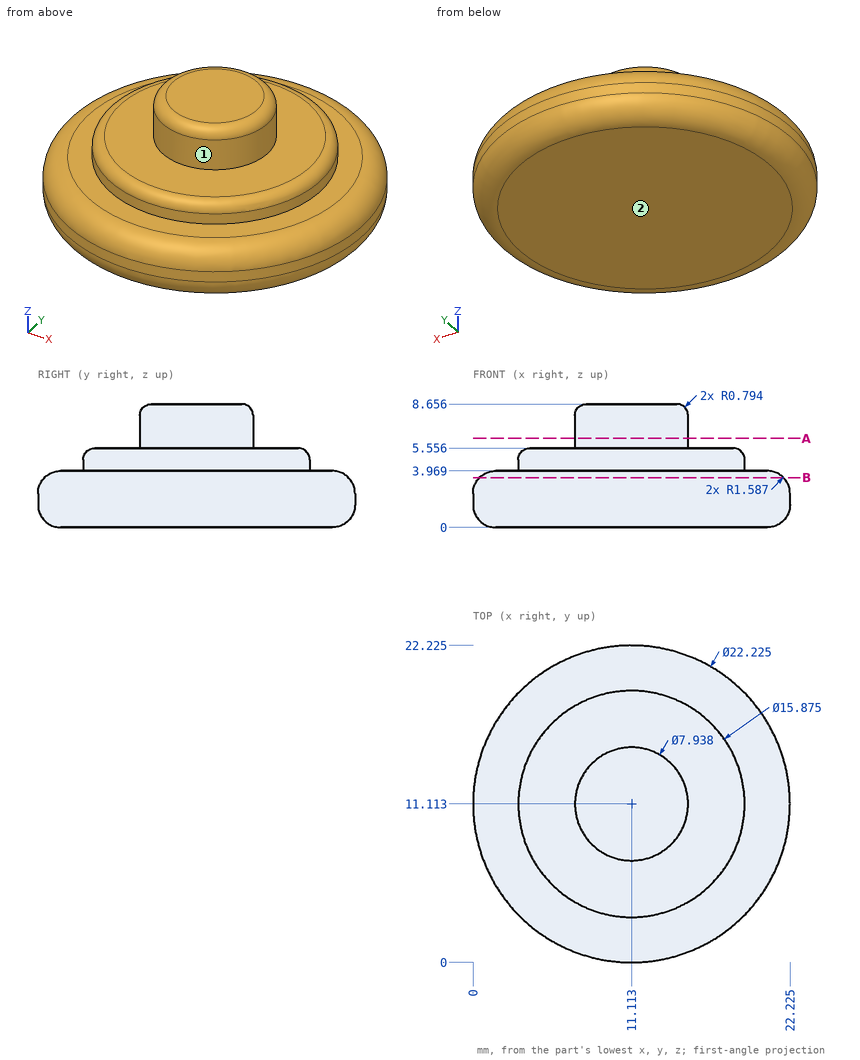
Input: dimensioned drawing with shaded views. Units: mm. Origin: part minimum x, y, z. A direction names the side the tool comes from. Coordinates: 2 decimals unless noted, no trailing zeros. Loops run counter-clockwise (first coordinate to the right, second up) from the corner with the lowest first, then second, coordinate; pieces in that order, holes last. Notation, with made-up numbers: (-14, 22) -> (13, 22) arc R21 ccw to (13, 45) -> close; hole circle Ø2 at (-11, 31.25). An arc over 180 degrees is marked (long way). Use a Markdown table: item, result. Add a question column.
(1) Section query B-B, the plane z = 3.5. Return loops of the section in (x, y), plus the area to 3 significant figures.
(2) Section query A-A, the plane z = 6.25. Return loops of the section in (x, y).
(3) Line query: line 1 along X through (y, z) = (11.25, 2.25) (1 decimal); line 2 along Z through (x, y) = (17.75, 6); line 3 along Z through (x, y) = (18.25, 12) (1 decimal). Output: solid intervals per line, ascending.
(4) Access query for the marked faces 1 and 2. Directions: +Z, -Z, +X, -X, +Y, -Y. A direction counts if a zero-diameter tool reaches every point of the face in a straight line with its end or side. Return the directions, or none.
(5) Pin query (flat end, axial travel): pin 1 Ø4.5 at (x, y) = (13, 14) entering from +Z; pin 2 Ø4 at (x, z) = (19, 1.5) entering from +Y (1 decimal); pin 3 Ø1.5 at (y, z) = (15, 2) entering from -X; pin 4 Ø4 at (y, z) = (5, 5) entering from +X (1 decimal). Return the tip coordinate at first contact, or that it passes through.
Answer:
| question | item | result |
|---|---|---|
| 1 | outline | circle Ø21.3 at (11.11, 11.11) |
| 1 | area | 356 mm^2 |
| 2 | outline | circle Ø7.94 at (11.11, 11.11) |
| 3 | line 1 | x = 0 to 22.2 |
| 3 | line 2 | z = 0 to 3.97 |
| 3 | line 3 | z = 0 to 5.6 |
| 4 | face 1 | +Z |
| 4 | face 2 | -Z, +X, -X, +Y, -Y |
| 5 | pin 1 | stops at z = 8.66 |
| 5 | pin 2 | stops at y = 20.5 |
| 5 | pin 3 | stops at x = 0.45 |
| 5 | pin 4 | stops at x = 20.7 |
